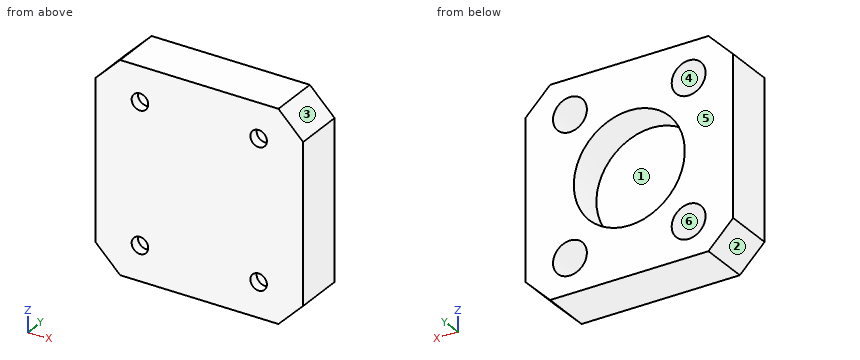
```python
from build123d import *

# Parameters (mm, degrees)
SKETCH1_W           = 42
SKETCH1_H           = 42
BOSS_EXTRUDE1_DEPTH = 10
SKETCH2_R           = 11.1
CUT_EXTRUDE1_DEPTH  = 7
CHAMFER1_SIZE       = 0.122185454
CHAMFER1_SIZE_2     = 7
SKETCH3_R           = 3.425
CUT_EXTRUDE2_DEPTH  = 8
CHAMFER2_SIZE       = 5
CUT_EXTRUDE3_REACH  = 32.757
SKETCH4_R           = 1.675


with BuildPart() as part:
    # Sketch1 → Boss-Extrude1 (new body)
    with BuildSketch(Plane(origin=(0, 0, 0), x_dir=(1, 0, 0), z_dir=(0, 1, 0))):
        Rectangle(SKETCH1_W, SKETCH1_H)
    extrude(amount=BOSS_EXTRUDE1_DEPTH)

    # Sketch2 → Cut-Extrude1 (cut)
    with BuildSketch(Plane(origin=(0, 10, 0), x_dir=(1, 0, 0), z_dir=(0, 1, 0))):
        with Locations(Location((0, 0, 0), (0, 0, 270))):
            Circle(SKETCH2_R)
    extrude(amount=-CUT_EXTRUDE1_DEPTH, mode=Mode.SUBTRACT)

    # Chamfer1
    # the kernel refuses this chamfer: 7, 0.122185454 mm, written as the material it takes off along each edge
    with BuildSketch(Plane(origin=(0, 10, 0), x_dir=(0, 0, 1), z_dir=(-1, 0, 0))) as chamfer1_piece_1_section:
        Polygon((11.1 + CHAMFER1_SIZE * 1.00000000407, 0), (11.1, -CHAMFER1_SIZE_2), (11.1, 0), align=None)
    chamfer1_piece_1 = revolve(axis=Axis((0, 10, 0), (0, 1, 0)), mode=Mode.PRIVATE)
    chamfer1_piece_1 = split(chamfer1_piece_1, bisect_by=Plane(origin=(0, 3, -11.117232441), z_dir=(0, 1, 0)), keep=Keep.TOP, mode=Mode.PRIVATE)
    add(chamfer1_piece_1, mode=Mode.SUBTRACT)

    # Sketch3 → Cut-Extrude2 (cut)
    with BuildSketch(Plane(origin=(0, 10, 0), x_dir=(1, 0, 0), z_dir=(0, 1, 0))):
        with Locations(Location((-12, 14, 0), (0, 0, 270))):
            Circle(SKETCH3_R)
        with Locations(Location((-12, -14, 0), (0, 0, 90))):
            Circle(SKETCH3_R)
        with Locations(Location((12, -14, 0), (0, 0, 270))):
            Circle(SKETCH3_R)
        with Locations(Location((12, 14, 0), (0, 0, 90))):
            Circle(SKETCH3_R)
    extrude(amount=-CUT_EXTRUDE2_DEPTH, mode=Mode.SUBTRACT)

    # Chamfer2
    chamfer2_edges = [part.edges().sort_by_distance(p)[0] for p in [
        (21, 5, 21),
        (-21, 5, 21),
        (-21, 5, -21),
        (21, 5, -21),
    ]]
    chamfer(chamfer2_edges, length=CHAMFER2_SIZE)

    # Sketch4 → Cut-Extrude3 (cut, up to next)
    with BuildSketch(Plane(origin=(0, 2, 0), x_dir=(1, 0, 0), z_dir=(0, 1, 0)), mode=Mode.PRIVATE) as cut_extrude3_sk1:
        with Locations(Location((-12, 14, 0), (0, 0, 270))):
            Circle(SKETCH4_R)
    cut_extrude3_tool1 = extrude(cut_extrude3_sk1.sketch, amount=-CUT_EXTRUDE3_REACH, mode=Mode.PRIVATE) & part.part
    # Sketch4 → Cut-Extrude3 (cut, up to next)
    with BuildSketch(Plane(origin=(0, 2, 0), x_dir=(1, 0, 0), z_dir=(0, 1, 0)), mode=Mode.PRIVATE) as cut_extrude3_sk2:
        with Locations(Location((12, 14, 0), (0, 0, 90))):
            Circle(SKETCH4_R)
    cut_extrude3_tool2 = extrude(cut_extrude3_sk2.sketch, amount=-CUT_EXTRUDE3_REACH, mode=Mode.PRIVATE) & part.part
    # Sketch4 → Cut-Extrude3 (cut, up to next)
    with BuildSketch(Plane(origin=(0, 2, 0), x_dir=(1, 0, 0), z_dir=(0, 1, 0)), mode=Mode.PRIVATE) as cut_extrude3_sk3:
        with Locations(Location((12, -14, 0), (0, 0, 270))):
            Circle(SKETCH4_R)
    cut_extrude3_tool3 = extrude(cut_extrude3_sk3.sketch, amount=-CUT_EXTRUDE3_REACH, mode=Mode.PRIVATE) & part.part
    # Sketch4 → Cut-Extrude3 (cut, up to next)
    with BuildSketch(Plane(origin=(0, 2, 0), x_dir=(1, 0, 0), z_dir=(0, 1, 0)), mode=Mode.PRIVATE) as cut_extrude3_sk4:
        with Locations(Location((-12, -14, 0), (0, 0, 90))):
            Circle(SKETCH4_R)
    cut_extrude3_tool4 = extrude(cut_extrude3_sk4.sketch, amount=-CUT_EXTRUDE3_REACH, mode=Mode.PRIVATE) & part.part
    add(cut_extrude3_tool1.solids().sort_by_distance((-12, 2, -14))[0], mode=Mode.SUBTRACT)
    add(cut_extrude3_tool2.solids().sort_by_distance((12, 2, -14))[0], mode=Mode.SUBTRACT)
    add(cut_extrude3_tool3.solids().sort_by_distance((12, 2, 14))[0], mode=Mode.SUBTRACT)
    add(cut_extrude3_tool4.solids().sort_by_distance((-12, 2, 14))[0], mode=Mode.SUBTRACT)


solid = part.part
```
The model under review builds one solid part; all positions refer to its coordinate system, in mm. Face numbers are marked on the shaded views. A direction names the side the tool comes from. Round coordinates to 2 decimals unless told otherwise and drop trailing zeros. Write each loop counter-clockwise with the first axis right and the second up, starting at its lowest first coordinate (ties: lowest second). Pieces come first, ordered by that corner, then holes.
(1) Mouldability with a two-part tool opening along X and no side actions: class the marked faces 1, 2, 3 and 4 as +X half, -X half, draft (parallel to the pull), parting line (faces both ways), or undercut.
(2) Insertion check: pin 1 (11 mm diameter, centred on x = -0.5, z = 5.5, fed in from +Y); pin 2 (5.5 mm diameter, centred on x = 12, z = 14, fed in from +Y); pin 3 (2 mm diameter, centred on x = 12, z = -14, fed in from -Y). Each pin has a flat end and moves straight along its axis. Give the tip position at first contact, or say it passes through.
(3) We need section C-C on y = 9. Give the boundary of the cut face in (x, z) (3 decimals), and give its area (3 significant figures).
(4) Wall thickness on L1, parallel to X at y = 1.5, z = -14 (3 decimals); L2, parallel to Z at x = 15, y = 2.5; L3, parallel to X at y = 5.25, z = 14 (3 decimals): over which ranges is each line inside the solid? List them lowest first.
(5) We need section A-A on z = -14. Give the boundary of the cut face in (x, y) (3 decimals), and give its area (3 significant figures).
(6) We need section B-B on x = 12. Give the boundary of the cut face in (y, z) (3 decimals).
(7) Machinability: for the marked faces 5 and 6, which of the approach directions +Z, -Z, +X, -X, +Y, -Y give a long, thin tool a straight path to every point of the face, cutting with its end or side? Answer none if there is none.
(8) We need section D-D on x = -18. Give the boundary of the cut face in (y, z).
Findings below:
1. face 1: undercut
1. face 2: -X half
1. face 3: +X half
1. face 4: undercut
2. pin 1: stops at y = 3
2. pin 2: stops at y = 2
2. pin 3: passes through
3. outline: (-21, -16) - (-16, -21) - (16, -21) - (21, -16) - (21, 16) - (16, 21) - (-16, 21) - (-21, 16) - close; hole circle Ø6.85 at (-12, -14); hole circle Ø6.85 at (-12, 14); hole circle Ø22.409 at (0, 0); hole circle Ø6.85 at (12, -14); hole circle Ø6.85 at (12, 14)
3. area: 1,170 mm2
4. L1: x = -21 to -13.675, -10.325 to 10.325, 13.675 to 21
4. L2: z = -21 to -15.65, -12.35 to 12.35, 15.65 to 21
4. L3: x = -21 to -15.425, -8.575 to 8.575, 15.425 to 21
5. outline: (-21, 0) - (-13.675, 0) - (-13.675, 2) - (-15.425, 2) - (-15.425, 10) - (-21, 10) - close; (-10.325, 0) - (10.325, 0) - (10.325, 2) - (8.575, 2) - (8.575, 10) - (-8.575, 10) - (-8.575, 2) - (-10.325, 2) - close; (13.675, 0) - (21, 0) - (21, 10) - (15.425, 10) - (15.425, 2) - (13.675, 2) - close
5. area: 297 mm2
6. outline: (0, -21) - (10, -21) - (10, -17.425) - (2, -17.425) - (2, -15.675) - (0, -15.675) - close; (0, -12.325) - (2, -12.325) - (2, -10.575) - (10, -10.575) - (10, 10.575) - (2, 10.575) - (2, 12.325) - (0, 12.325) - close; (0, 15.675) - (2, 15.675) - (2, 17.425) - (10, 17.425) - (10, 21) - (0, 21) - close
7. face 5: +Z, -Z, +X, -X, +Y
7. face 6: +Y
8. outline: (0, -19) - (10, -19) - (10, 19) - (0, 19) - close
